Autodesk Inventor part; units mm, degrees
ref_plane "YZ Plane" through (0, 0, 0) normal (1, 0, 0) x (0, 1, 0)
ref_plane "XZ Plane" through (0, 0, 0) normal (0, 1, 0) x (-1, 0, 0)
ref_plane "XY Plane" through (0, 0, 0) normal (0, 0, 1) x (1, 0, 0)
sketch "Sketch1" plane through (0, 0, 0) normal (0, 1, 0) x (-1, 0, 0)
  line L0 (-400, 600) -> (400, 600)
  line L1 (400, 600) -> (400, -600)
  line L2 (400, -600) -> (-400, -600)
  line L3 (-400, -600) -> (-400, 600)
  line L4 (-400, 600) -> (400, -600) construction
  line L5 (400, 600) -> (-400, -600) construction
  point P0 (0, 0)
  dimension "d0" = 800
  dimension "d1" = 1200
extrude "Extrusion1" add sketch "Sketch1" along normal blind 235
sketch "Sketch2" plane through (0, 0, 0) normal (0, -1, 0) x (1, 0, 0)
  line L0 (200, 400) -> (-200, 400)
  line L1 (-200, 400) -> (-200, 420)
  line L2 (-200, 420) -> (200, 420)
  line L3 (200, 420) -> (200, 400)
  line L4 (200, 400) -> (-200, 420) construction
  line L5 (-200, 400) -> (200, 420) construction
  line L6 (200, -420) -> (-200, -420)
  line L7 (-200, -420) -> (-200, -400)
  line L8 (-200, -400) -> (200, -400)
  line L9 (200, -400) -> (200, -420)
  line L10 (200, -420) -> (-200, -400) construction
  line L11 (-200, -420) -> (200, -400) construction
  line L12 (400, -600) -> (-400, -600)
  line L13 (400, 600) -> (400, -600)
  point P0 (0, 0)
  point P1 (0, 410)
  point P2 (0, -410)
  dimension "d4" = 400
  dimension "d5" = 20
  dimension "d6" = 400
  dimension "d7" = 20
  dimension "d9" = 800
  dimension "d10" = 180
  dimension "d11" = 200
  dimension "d12" = 200
extrude "Extrusion2" add sketch "Sketch2" along normal blind 35
sketch "Sketch3" plane through (-200, 0, 420) normal (0, 0, 1) x (1, 0, 0)
  line L0 (10, -10) -> (390, -10)
  line L1 (390, -10) -> (390, -25)
  line L2 (390, -25) -> (10, -25)
  line L3 (10, -25) -> (10, -10)
  line L4 (10, -10) -> (390, -25) construction
  line L5 (390, -10) -> (10, -25) construction
  line L6 (400, -35) -> (0, -35)
  line L7 (400, 0) -> (400, -35)
  point P0 (200, 0)
  point P1 (200, -17.5)
  dimension "d15" = 380
  dimension "d16" = 15
  dimension "d17" = 10
  dimension "d18" = 10
extrude "Extrusion3" cut sketch "Sketch3" against normal blind 1000
fillet "Fillet1" radius 10 8 edges at (0, 0, 600) (400, 0, 0) (400, 117.5, 600) (-400, 117.5, 600) (-400, 0, 0) (-400, 117.5, -600) (0, 0, -600) (400, 117.5, -600)
sketch "Sketch8" plane through (400, 10, 590) normal (1, 0, 0) x (0, 0, -1)
  line L0 (940, 225) -> (940, 25) construction
  circle A0 centre (940, 125) radius 50
  line L1 (0, 225) -> (1180, 225)
  line L2 (0, -10) -> (1180, -10)
  line L3 (1190, 0) -> (1190, 225)
  line L4 (200, 80) -> (330, 80)
  line L5 (330, 80) -> (330, 170)
  line L6 (330, 170) -> (200, 170)
  line L7 (200, 170) -> (200, 80)
  line L8 (200, 80) -> (330, 170) construction
  line L9 (330, 80) -> (200, 170) construction
  line L10 (940, 125) -> (0, 125) construction
  line L11 (0, 0) -> (0, 225)
  point P0 (590, -10)
  point P1 (265, 125)
  point P2 (265, 125)
  dimension "d39" = 100
  dimension "d40" = 35
  dimension "d41" = 250
  dimension "d44" = 130
  dimension "d45" = 90
  dimension "d46" = 200
extrude "Extrusion7" cut sketch "Sketch8" against normal blind 50
sketch "Sketch9" plane through (0, 235, 0) normal (0, 1, 0) x (1, 0, 0)
  line L0 (-380, -550) -> (380, -550)
  line L1 (380, -550) -> (380, 550)
  line L2 (380, 550) -> (-380, 550)
  line L3 (-380, 550) -> (-380, -550)
  line L4 (-380, -550) -> (380, 550) construction
  line L5 (380, -550) -> (-380, 550) construction
  line L6 (400, -590) -> (400, 590)
  line L7 (390, 600) -> (-390, 600)
  line L8 (-350, -580) -> (350, -580)
  line L9 (350, -580) -> (350, 580)
  line L10 (350, 580) -> (-350, 580)
  line L11 (-350, 580) -> (-350, -580)
  line L12 (-350, -580) -> (350, 580) construction
  line L13 (350, -580) -> (-350, 580) construction
  point P0 (0, 0)
  point P1 (-350, -550)
  point P2 (350, -550)
  point P3 (350, 550)
  point P4 (-350, 550)
  dimension "d47" = 20
  dimension "d48" = 50
  dimension "d49" = 50
  dimension "d50" = 20
extrude "Extrusion8" cut sketch "Sketch9" against normal blind 200
properties part number "señales_carcasa_x10"
Work out the finished part from the listing and answer in its coordinate system (mm). A direction names the side the tool comes from. Give positions to 0.01 mm unless a question says otherwise; leave off trailing zeros. Order: outer loops, then holes, each group sorted by start corner. A loop starts at its lowest first (then second) coordinate and runs counter-clockwise, first axis right, second up. Notation, with made-up numbers: (-20, 75) - (3, 75) arc R32 cw to (3, 114) - close; hole circle Ø4 at (-8, -2). An arc over 180 degrees is marked (long way). Answer as CSV lines item,"result". Start each with the question number.
Q1. The part is cut by section D-D (x = -311.5). Write down the section's boundary in (y, z), then the cut area to 3 significant figures.
Q2. The part is cut by section C-C (z = -350). Write down the section's boundary in (x, y), then the cut area to 3 significant figures.
Q3. Given pin 1 Ø3 at (x, z) = (17.5, 158.5) entering from +Y; pin 2 Ø2 at (x, y) = (-56, 3) entering from -Z; pin 3 Ø16.5 at (y, z) = (-20, -411.5) entering from -X, each flat-ended and moving along its own axis, determine where each tip first touches the part or whether it passes through.
Q4. The part is cut by section A-A (x = -74.5). Write down the section's boundary in (y, z), then the cut area to 3 significant figures.
Q5. Find the intervals of material crossed by L1, parallel to Z at x = -307.5, y = 113; L2, parallel to Y at x = 388, z = -350; L3, parallel to X at y = 170, z = -210, in increasing order. Write a range as [from, to].
Q6. For faces 4 (the face through (5, 136, -580)), 5 (the face through (3, -9, -420)), 6 (the face through (-3, -9, 420)), 7 (the face through (-383, 235, 181)), 8 (the face through (390.14, 115.85, -396.187)), determine the directions among +Z, -Z, +X, -X, +Y, -Y from which every point of the face is accessible in a straight line to the end or side of a thin tool.
Q7. The mould has two halves that part along X. Classify faces 1 (the face through (-380, 136, -8)), 2 (the face through (3, -9, 400)), 3 (the face through (-365, 136, 550)): +X half, -X half, draft (parallel to the pull), parting line (faces both ways), or undercut.
Q8. The part is cut by section B-B (y = 135). Write down the section's boundary in (x, z).
Check result:
1,outline,"(0, -590) arc R10 ccw to (10, -600) - (235, -600) - (235, -580) - (35, -580) - (35, 580) - (235, 580) - (235, 600) - (10, 600) arc R10 ccw to (0, 590) - close"
1,area,"50,000 mm²"
2,outline,"(-400, 10) arc R10 ccw to (-390, 0) - (390, 0) arc R10 ccw to (400, 10) - (400, 85) - (380, 85) - (380, 35) - (-380, 35) - (-380, 235) - (-400, 235) - close; (380, 185) - (400, 185) - (400, 235) - (380, 235) - close"
2,area,"34,000 mm²"
3,pin 1,"stops at y = 35"
3,pin 2,"stops at z = -598"
3,pin 3,"stops at x = -200"
4,outline,"(-35, -420) - (-25, -420) - (-25, -400) - (-35, -400) - close; (-35, 400) - (-25, 400) - (-25, 420) - (-35, 420) - close; (-10, -420) - (0, -420) - (0, -590) arc R10 ccw to (10, -600) - (235, -600) - (235, -580) - (35, -580) - (35, 580) - (235, 580) - (235, 600) - (10, 600) arc R10 ccw to (0, 590) - (0, 420) - (-10, 420) - (-10, 400) - (0, 400) - (0, -400) - (-10, -400) - close"
4,area,"50,800 mm²"
5,L1,"z = [-600, -580], [580, 600]"
5,L2,"y = [0, 85], [185, 235]"
5,L3,"x = [-400, -380], [380, 400]"
6,face 4,"+Y"
6,face 5,"-Z, +X, -X, -Y"
6,face 6,"+Z, +X, -X, -Y"
6,face 7,"+Z, -Z, +X, -X, +Y"
6,face 8,"+X"
7,face 1,"undercut"
7,face 2,"draft"
7,face 3,"undercut"
8,outline,"(-400, -590) arc R10 ccw to (-390, -600) - (390, -600) arc R10 ccw to (400, -590) - (400, -400) - (380, -400) - (380, -550) - (350, -550) - (350, -580) - (-350, -580) - (-350, -550) - (-380, -550) - (-380, 550) - (-350, 550) - (-350, 580) - (350, 580) - (350, 550) - (380, 550) - (380, 390) - (400, 390) - (400, 590) arc R10 ccw to (390, 600) - (-390, 600) arc R10 ccw to (-400, 590) - close; (380, -300) - (400, -300) - (400, 260) - (380, 260) - close"
